Source: three-view drawing plus pictorial views. Frame: mm from the lowest corner of the part. Round coordinates to 2 decimals unless told otherwise and drop trailing zeros. Order: outer loops, then holes, each group sorted by start corner. A loop starts at its lowest first (then second) coordinate and runs counter-clockwise, first axis right, second up. Notation, with made-up numbers: (9, 85) -> (49, 85) arc R30 cw to (49, 118) -> close; hole circle Ø11 at (26, 78). An arc over 180 degrees is marked (long way). Answer as CSV lines item,"result".
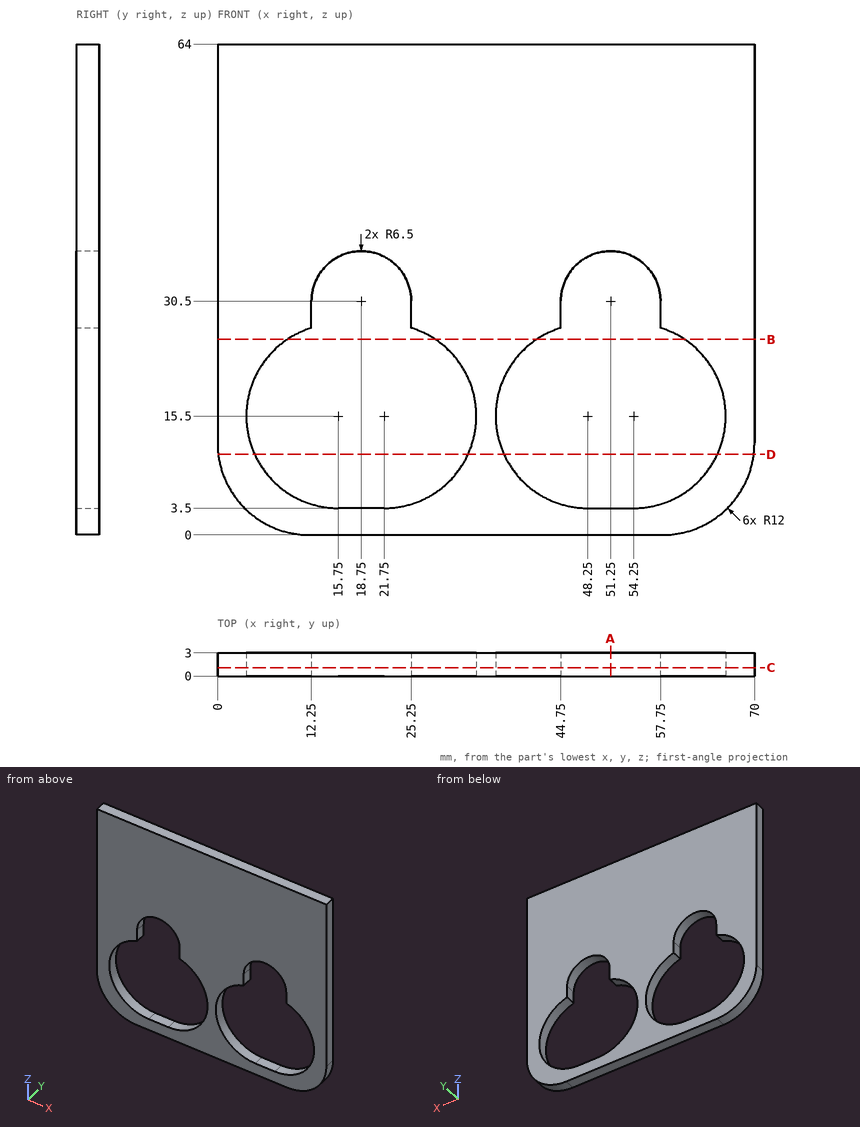
1. Line query: L1, parallel to X at y = 2, z = 28.5; L2, parallel to X at y = 2.6, z = 15.5; L3, parallel to Z at x = 46.5, y = 1.25. Output: solid intervals per line, ascending. Write a range as [from, to].
Results below:
L1,"[0, 12.25], [25.25, 44.75], [57.75, 70]"
L2,"[0, 3.75], [33.75, 36.25], [66.25, 70]"
L3,"[0, 3.63], [34.94, 64]"
2. Section query C-C on y = 1.1. Return loops of the section in (x, z), and give its area (3 significant figures).
Results below:
outline,"(0, 12) arc R12 ccw to (12, 0) -> (58, 0) arc R12 ccw to (70, 12) -> (70, 64) -> (0, 64) -> close; hole (12.25, 26.98) arc R12 ccw to (15.75, 3.5) -> (21.75, 3.5) arc R12 ccw to (25.25, 26.98) -> (25.25, 30.5) arc R6.5 ccw to (12.25, 30.5) -> close; hole (44.75, 26.98) arc R12 ccw to (48.25, 3.5) -> (54.25, 3.5) arc R12 ccw to (57.75, 26.98) -> (57.75, 30.5) arc R6.5 ccw to (44.75, 30.5) -> close"
area,"3,010 mm2"
3. Section query B-B on z = 25.5. Return loops of the section in (x, y).
Results below:
outline,"(0, 0) -> (9.12, 0) -> (9.12, 3) -> (0, 3) -> close; (28.38, 0) -> (41.62, 0) -> (41.62, 3) -> (28.38, 3) -> close; (60.88, 0) -> (70, 0) -> (70, 3) -> (60.88, 3) -> close"
4. Section query A-A on x = 51.25. Return loops of the section in (y, z).
Results below:
outline,"(0, 0) -> (3, 0) -> (3, 3.5) -> (0, 3.5) -> close; (0, 37) -> (3, 37) -> (3, 64) -> (0, 64) -> close"
5. Section query D-D on z = 10.5. Return loops of the section in (x, y), and give its area (3 significant figures).
Results below:
outline,"(0.09, 0) -> (4.84, 0) -> (4.84, 3) -> (0.09, 3) -> close; (32.66, 0) -> (37.34, 0) -> (37.34, 3) -> (32.66, 3) -> close; (65.16, 0) -> (69.91, 0) -> (69.91, 3) -> (65.16, 3) -> close"
area,"42.5 mm2"
